Verification items for this drawing (mm, ordinates from the low corner). A direction names the side the tool comes from. Round coordinates to 2 decimals unless told otherwise and drop trailing zeros. Order: outer loops, then holes, each group sorted by start corner. A loop starts at its lowest first (then second) coordinate and runs counter-clockwise, first axis right, second up. Notation, with made-up numbers: M 62,79.25 L 97,79.25 A31 cw 97,112.25 Z; hole C 6,-39 d4. An arc over 180 degrees is marked long. Return JSON: item names as keys, results as strings. Group by question number.
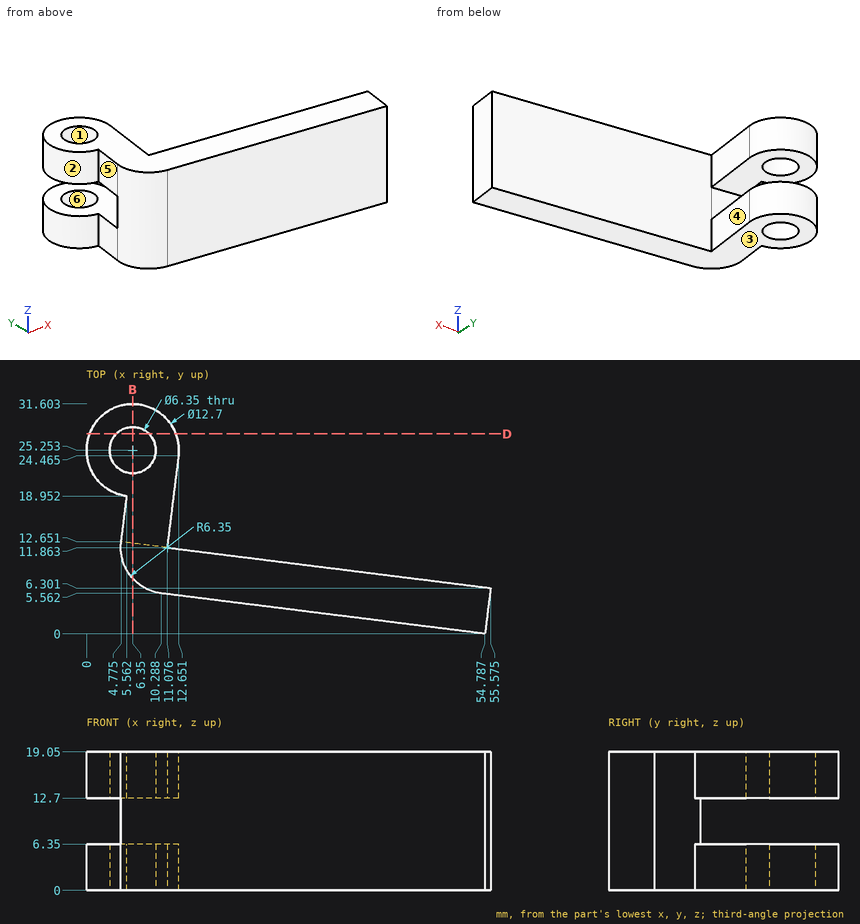
1. Thickness scan on line 1 along Z through (x, y) = (11.5, 25.5); line 2 along X through (y, z) = (27, 4) (1 decimal); line 3 along Y through (x, z) = (6.35, 2) (1 decimal). Record the ranges inside material, lowest first. Write a range as from..to.
2. Draft check along X on the marked faces 1, 2 and 3. Enter one of: +X half, -X half, draft (parallel to the pull), parting line (faces both ways), or undercut.
3. Cross-section at B-B (x = 6.35). Enter the section's corners in (y, z), plus the area to 3 significant figures.
4. Access from +Z, -Z, +X, -X, +Y, -Y to the whole of each face (thin tool, end or side, straight path). Record for the marked faces 4, 5 and 6.
5. Cross-section at D-D (y = 27.5). Enter the section's corners in (x, z).
6. Go/stop test with flat-tipped pins: pin 1 (6.5 mm diameter, centred on x = 5.5, y = 26.5, fed in from -Z); pin 2 (2 mm diameter, centred on x = 39.5, z = 10, fed in from +Y) (1 decimal); pin 3 (12 mm diameter, centred on x = 36, y = 19.5, fed in from -Z); pin 4 (3 mm diameter, centred on x = 39.5, z = 17, fed in from -Y). Record where each tip stops, or that it passes through.
Computed:
{
 "1": {"line 1": "z = 0..6.35, 12.7..19.05", "line 2": "x = 0.2..3.7, 9..12.5", "line 3": "y = 7.6..22.1, 28.4..31.6"},
 "2": {"face 1": "undercut", "face 2": "parting line", "face 3": "draft"},
 "3": {"outline": "M 7.62,0 L 22.08,0 L 22.08,6.35 L 12.45,6.35 L 12.45,12.7 L 22.08,12.7 L 22.08,19.05 L 7.62,19.05 Z; M 28.43,0 L 31.6,0 L 31.6,6.35 L 28.43,6.35 Z; M 28.43,12.7 L 31.6,12.7 L 31.6,19.05 L 28.43,19.05 Z", "area": "255 mm²"},
 "4": {"face 4": "+Z, -Z, +X", "face 5": "+Z, -Z, -X", "face 6": "+Z, -Z"},
 "5": {"outline": "M 0.41,0 L 4.11,0 L 4.11,6.35 L 0.41,6.35 Z; M 0.41,12.7 L 4.11,12.7 L 4.11,19.05 L 0.41,19.05 Z; M 8.59,0 L 12.29,0 L 12.29,6.35 L 8.59,6.35 Z; M 8.59,12.7 L 12.29,12.7 L 12.29,19.05 L 8.59,19.05 Z"},
 "6": {"pin 1": "stops at z = 0", "pin 2": "stops at y = 8.4", "pin 3": "passes through", "pin 4": "stops at y = 1.72"}
}
